from build123d import *

# Parameters (mm, degrees)
SKETCH1_W           = 30.5
SKETCH1_H           = 13.75
BOSS_EXTRUDE2_DEPTH = 1.15
BOSS_EXTRUDE4_DEPTH = 5
BOSS_EXTRUDE5_DEPTH = 0.1
CUT_EXTRUDE1_DEPTH  = 0.05
SKETCH6_W           = 1.5
SKETCH6_H           = 0.75
BOSS_EXTRUDE6_DEPTH = 0.05
SKETCH7_R           = 0.5
CUT_EXTRUDE2_DEPTH  = 2.25
SKETCH8_W           = 4
SKETCH8_H           = 5
BOSS_EXTRUDE7_DEPTH = 1.5
FILLET1_R           = 0.5
SKETCH9_W           = 1.5
SKETCH9_H           = 0.495696311
BOSS_EXTRUDE8_DEPTH = 0.5


with BuildPart() as part:
    # Sketch1 → Boss-Extrude2 (new body)
    with BuildSketch(Plane(origin=(0, 0, 0), x_dir=(1, 0, 0), z_dir=(0, 1, 0))):
        with Locations((-7.383484163, -5.632918552)):
            Rectangle(SKETCH1_W, SKETCH1_H)
    extrude(amount=BOSS_EXTRUDE2_DEPTH)

    # Sketch3 → Boss-Extrude4 (add)
    with BuildSketch(Plane(origin=(0, 1.15, 0), x_dir=(1, 0, 0), z_dir=(0, 1, 0))):
        Polygon((-9.204551975, -5.972384646), (-5.669018069, -9.507918552), (-2.133484163, -5.972384646), (-5.669018069, -2.43685074), align=None)
    extrude(amount=BOSS_EXTRUDE4_DEPTH)

    # Sketch4 → Boss-Extrude5 (add)
    with BuildSketch(Plane(origin=(0, 6.15, 0), x_dir=(1, 0, 0), z_dir=(0, 1, 0))):
        with BuildLine():
            ThreePointArc((-6.919018069, -5.972384646), (-5.669018069, -7.222384646), (-4.419018069, -5.972384646))
            Line((-4.419018069, -5.972384646), (-6.919018069, -5.972384646))
        make_face()
        with BuildLine():
            Line((-6.919018069, -5.972384646), (-4.419018069, -5.972384646))
            ThreePointArc((-4.419018069, -5.972384646), (-5.669018069, -4.722384646), (-6.919018069, -5.972384646))
        make_face()
    extrude(amount=BOSS_EXTRUDE5_DEPTH)

    # Sketch5 → Cut-Extrude1 (cut)
    with BuildSketch(Plane(origin=(0, 6.25, 0), x_dir=(1, 0, 0), z_dir=(0, 1, 0))):
        with BuildLine():
            Line((-6.919018069, -5.972384646), (-4.419018069, -5.972384646))
            ThreePointArc((-4.419018069, -5.972384646), (-4.425347878, -5.846748444), (-4.444273197, -5.722384646))
            Line((-4.444273197, -5.722384646), (-6.89376294, -5.722384646))
            ThreePointArc((-6.89376294, -5.722384646), (-6.91268826, -5.846748444), (-6.919018069, -5.972384646))
        make_face()
        with BuildLine():
            ThreePointArc((-4.444273197, -6.222384646), (-4.425347878, -6.098020849), (-4.419018069, -5.972384646))
            Line((-4.419018069, -5.972384646), (-6.919018069, -5.972384646))
            ThreePointArc((-6.919018069, -5.972384646), (-6.91268826, -6.098020849), (-6.89376294, -6.222384646))
            Line((-6.89376294, -6.222384646), (-4.444273197, -6.222384646))
        make_face()
    extrude(amount=-CUT_EXTRUDE1_DEPTH, mode=Mode.SUBTRACT)

    # Sketch6 → Boss-Extrude6 (add)
    with BuildSketch(Plane(origin=(0, 1.15, 0), x_dir=(1, 0, 0), z_dir=(0, 1, 0))):
        with BuildLine():
            ThreePointArc((-3.003484163, -11.257918552), (-2.253484163, -12.007918552), (-1.503484163, -11.257918552))
            Line((-1.503484163, -11.257918552), (-3.003484163, -11.257918552))
        make_face()
        with BuildLine():
            Line((-3.003484163, -11.257918552), (-1.503484163, -11.257918552))
            ThreePointArc((-1.503484163, -11.257918552), (-2.253484163, -10.507918552), (-3.003484163, -11.257918552))
        make_face()
        with BuildLine():
            ThreePointArc((-0.463484163, -11.257918552), (0.286515837, -12.007918552), (1.036515837, -11.257918552))
            Line((1.036515837, -11.257918552), (-0.463484163, -11.257918552))
        make_face()
        with BuildLine():
            Line((-0.463484163, -11.257918552), (1.036515837, -11.257918552))
            ThreePointArc((1.036515837, -11.257918552), (0.286515837, -10.507918552), (-0.463484163, -11.257918552))
        make_face()
        with BuildLine():
            ThreePointArc((2.076515837, -11.257918552), (2.826515837, -12.007918552), (3.576515837, -11.257918552))
            Line((3.576515837, -11.257918552), (2.076515837, -11.257918552))
        make_face()
        with BuildLine():
            Line((2.076515837, -11.257918552), (3.576515837, -11.257918552))
            ThreePointArc((3.576515837, -11.257918552), (2.826515837, -10.507918552), (2.076515837, -11.257918552))
        make_face()
        with Locations((5.366515837, -10.882918552)):
            Rectangle(SKETCH6_W, SKETCH6_H)
        with Locations((5.366515837, -11.632918552)):
            Rectangle(SKETCH6_W, SKETCH6_H)
        with BuildLine():
            ThreePointArc((-17.083484163, -11.257918552), (-16.333484163, -12.007918552), (-15.583484163, -11.257918552))
            Line((-15.583484163, -11.257918552), (-17.083484163, -11.257918552))
        make_face()
        with BuildLine():
            Line((-17.083484163, -11.257918552), (-15.583484163, -11.257918552))
            ThreePointArc((-15.583484163, -11.257918552), (-16.333484163, -10.507918552), (-17.083484163, -11.257918552))
        make_face()
        with BuildLine():
            ThreePointArc((-20.383484163, -11.257918552), (-19.633484163, -12.007918552), (-18.883484163, -11.257918552))
            Line((-18.883484163, -11.257918552), (-20.383484163, -11.257918552))
        make_face()
        with BuildLine():
            Line((-20.383484163, -11.257918552), (-18.883484163, -11.257918552))
            ThreePointArc((-18.883484163, -11.257918552), (-19.633484163, -10.507918552), (-20.383484163, -11.257918552))
        make_face()
        with BuildLine():
            ThreePointArc((-22.133484163, -11.257918552), (-21.383484163, -12.007918552), (-20.633484163, -11.257918552))
            Line((-20.633484163, -11.257918552), (-22.133484163, -11.257918552))
        make_face()
        with BuildLine():
            Line((-22.133484163, -11.257918552), (-20.633484163, -11.257918552))
            ThreePointArc((-20.633484163, -11.257918552), (-21.383484163, -10.507918552), (-22.133484163, -11.257918552))
        make_face()
    boss_extrude6 = extrude(amount=BOSS_EXTRUDE6_DEPTH)

    # Mirror1: Boss-Extrude6 across plane
    add(boss_extrude6.mirror(Plane.ZX.offset(0.575)))

    # Sketch7 → Cut-Extrude2 (cut, through all)
    with BuildSketch(Plane(origin=(0, 1.2, 0), x_dir=(1, 0, 0), z_dir=(0, 1, 0))):
        with Locations((-21.383484163, -11.257918552)):
            Circle(SKETCH7_R)
        with Locations((-19.633484163, -11.257918552)):
            Circle(SKETCH7_R)
        with Locations((-16.333484163, -11.257918552)):
            Circle(SKETCH7_R)
        with Locations((-2.253484163, -11.257918552)):
            Circle(SKETCH7_R)
        with Locations((0.286515837, -11.257918552)):
            Circle(SKETCH7_R)
        with Locations((2.826515837, -11.257918552)):
            Circle(SKETCH7_R)
        with Locations((5.366515837, -11.257918552)):
            Circle(SKETCH7_R)
    extrude(amount=-CUT_EXTRUDE2_DEPTH, mode=Mode.SUBTRACT)

    # Sketch8 → Boss-Extrude7 (add)
    with BuildSketch(Plane(origin=(0, 1.15, 0), x_dir=(1, 0, 0), z_dir=(0, 1, 0))):
        with Locations((3.366515837, -1.507918552)):
            Rectangle(SKETCH8_W, SKETCH8_H)
    extrude(amount=BOSS_EXTRUDE7_DEPTH)

    # Fillet1
    fillet1_edges = [part.edges().sort_by_distance(p)[0] for p in [
        (5.366515837, 2.65, 1.507918552),
        (3.366515837, 2.65, -0.992081448),
        (1.366515837, 2.65, 1.507918552),
        (3.366515837, 2.65, 4.007918552),
    ]]
    fillet(fillet1_edges, radius=FILLET1_R)

    # Sketch9 → Boss-Extrude8 (add)
    with BuildSketch(Plane(origin=(0, 1.15, 0), x_dir=(1, 0, 0), z_dir=(0, 1, 0))):
        with Locations((6.116515837, -0.923867938)):
            Rectangle(SKETCH9_W, SKETCH9_H)
        with Locations((6.116515837, -2.091969167)):
            Rectangle(SKETCH9_W, SKETCH9_H)
        with Locations((6.116515837, -3.260070397)):
            Rectangle(SKETCH9_W, SKETCH9_H)
        with Locations((6.116515837, 0.244233293)):
            Rectangle(SKETCH9_W, SKETCH9_H)
        with Locations((0.616515837, -3.260070397)):
            Rectangle(SKETCH9_W, SKETCH9_H)
        with Locations((0.616515837, -2.091969167)):
            Rectangle(SKETCH9_W, SKETCH9_H)
        with Locations((0.616515837, -0.923867938)):
            Rectangle(SKETCH9_W, SKETCH9_H)
        with Locations((0.616515837, 0.244233293)):
            Rectangle(SKETCH9_W, SKETCH9_H)
    extrude(amount=BOSS_EXTRUDE8_DEPTH)


solid = part.part
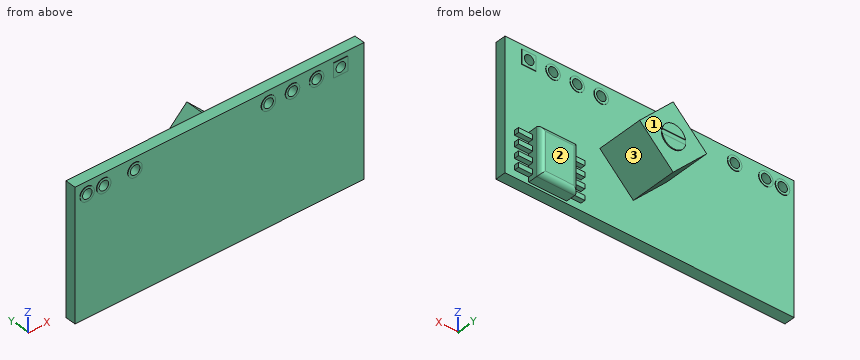
Can you work these out from the model? Positions are in its coordinate system, mm. Face numbers are marked on the shaded views. A direction names the side the tool comes from. Give positions to 0.01 mm unless a question says otherwise; leave off trailing zeros. Order: outer loops, then holes, each group sorted by start corner. A loop starts at its lowest first (then second) coordinate and runs counter-clockwise, first axis right, second up. Notation, with made-up numbers: M -36,54 L 9,54 A12 cw 9,68 Z; hole C -33.75,57 d11. An arc over 180 degrees is marked long. Use a Markdown table: item, result. Add a question column.
Item 1: Suppose I cut it at C-C (x = -11.5). List the corners of the cut face in (y, z) for me, then the cut area to 3 significant figures.
Item 2: If I drill on L1, parallel to Y at x = -10.5, z = 6.5; L2, parallel to Y at x = -4.5, z = 8.25; L3, parallel to Z at x = -4, y = 2, over which ranges is the centre line in solid material (lowest first)? Write a range as [from, to].
Item 3: Suppose I cut it at A-A (x = 3). List the corners of the cut face in (y, z) for me.
Item 4: Suppose I cut it at B-B (y = 3.25). List the corners of the cut face in (x, z) for me.
Item 5: Will these pins go through, and if not, where does the flat tip stop? pin 1 (0.5 mm diameter, centred on y = 1.5, z = -0.5, fed in from +X); pin 2 (8 mm diameter, centred on x = 1, z = 9.5, fed in from -Y); pin 3 (0.8 mm diameter, centred on x = 5.5, z = 11, fed in from +Y); pin 4 (0.6 mm diameter, centred on x = 6, y = 1.5, fed in from +Z).
Item 6: For the marked faces 1, 2 and 3, which set-ups out of +Z, -Z, +X, -X, +Y, -Y let a thin tool reach every point of the face, with its end or its side?
Answer sheet:
| question | item | result |
|---|---|---|
| 1 | outline | M 0,-1.24 L 1.15,-1.24 L 1.15,12.51 L 0,12.51 Z |
| 1 | area | 15.8 mm² |
| 2 | L1 | y = [0, 1.15] |
| 2 | L2 | y = [0, 6.15] |
| 2 | L3 | z = [4.11, 7.84] |
| 3 | outline | M -0.05,10.53 L 0,10.53 L 0,-1.24 L 1.15,-1.24 L 1.15,-0.99 L 2.15,-0.99 A0.5 ccw 2.65,-0.49 L 2.65,3.51 A0.5 ccw 2.15,4.01 L 1.15,4.01 L 1.15,10.53 L 1.2,10.53 L 1.2,10.79 L -0.05,10.79 Z; M -0.05,11.73 L 1.2,11.73 L 1.2,11.99 L 1.15,11.99 L 1.15,12.51 L 0,12.51 L 0,11.99 L -0.05,11.99 Z |
| 4 | outline | M -9.2,5.97 L -5.67,2.44 L -2.13,5.97 L -5.67,9.51 Z |
| 5 | pin 1 | stops at x = 6.87 |
| 5 | pin 2 | stops at y = -0.05 |
| 5 | pin 3 | stops at y = 1.2 |
| 5 | pin 4 | stops at z = 3.51 |
| 6 | face 1 | +Y |
| 6 | face 2 | +Z, -Z, +X, +Y |
| 6 | face 3 | -Z, +Y |
